Verification items for the finished model (mm, model axes). Face numbers are marked on the shaded views. A direction names the side the tool comes from. Round coordinates to 2 decimals unless told otherwise and drop trailing zeros. Order: outer loops, then holes, each group sorted by start corner. A loop starts at its lowest first (then second) coordinate and runs counter-clockwise, first axis right, second up. Notation, with made-up numbers: (40.25, -38.75) -> (60.25, -38.75) arc R15 cw to (60.25, -31.75) -> close; hole circle Ø2 at (40.25, 18.5). An arc over 180 degrees is marked (long way). Return JSON: item names as keys, results as strings. Group by question number.
Item 1: Access from +Z, -Z, +X, -X, +Y, -Y to the whole of each face (thin tool, end or side, straight path). Record for the marked faces 1, 2 and 3.
Item 2: Draft check along X on the marked faces 4, 5, 6 and 7. Enter one of: pulls with the +X half, pulls with the -X half, needs draft (parallel to the pull), parting line crosses it, or undercut.
Item 3: Sectioned sample at D-D on x = -6.5. Record the cut outline in (y, z), plus the area to 3 significant figures.
Item 4: Scan lines: probe 1 along X at (y, z) = (2, 21); probe 2 along Z at (x, y) = (-6, 4); probe 3 along Z at (x, y) = (8.5, 3.75). Record each from-to range of solid material in increasing order. Write a range as from..to.
Item 5: Sectioned sample at A-A on x = 6. Record the cut outline in (y, z), plus the area to 3 significant figures.
Item 6: Sectioned sample at B-B on y = -1.25. Record the cut outline in (x, z), plus the area to 3 significant figures.
Item 7: Sectioned sample at C-C on x = -3. Record the cut outline in (y, z).
Item 8: Depth check by flat-ended pin: pin 1 Ø2 at (y, z) = (0, 18) entering from +X; pin 2 Ø3.5 at (y, z) = (1, 17.5) entering from -X; pin 3 Ø9 at (x, z) = (-3.5, 4.5) entering from +Y; pin 4 Ø3 at (x, y) = (16, 0.5) entering from +Z. Enter the tip coordinate at first touch or a pass-through.
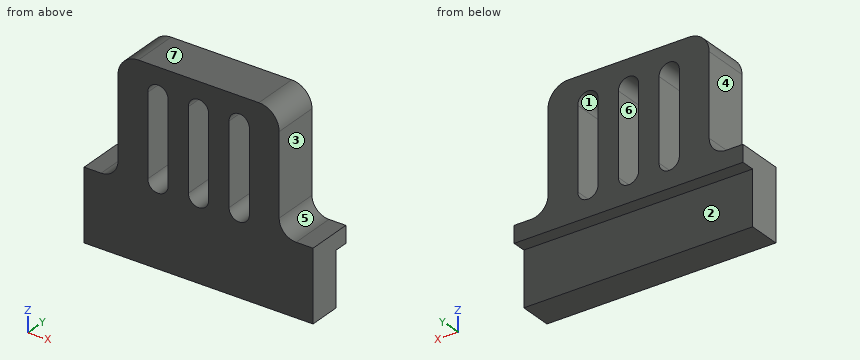
```python
from build123d import *

# Parameters (mm, degrees)
SKETCH_1_W          = 33.8
SKETCH_1_H          = 4.8
EXTRUDE_1_DEPTH     = 28
SKETCH_2_W          = 33.8
SKETCH_2_H          = 2
EXTRUDE_2_DEPTH     = 20
CUT_EXTRUDE_1_DEPTH = 34.404341035
SKETCH_4_W          = 5
SKETCH_4_H          = 17.5
CUT_EXTRUDE_2_DEPTH = 34.404341035
FILLET_1_R          = 3
FILLET_3_R          = 2.5


with BuildPart() as part:
    # 草圖1 → 填料-伸長1 (new body)
    with BuildSketch(Plane.XY):
        Rectangle(SKETCH_1_W, SKETCH_1_H)
    extrude(amount=EXTRUDE_1_DEPTH)

    # 草圖2 → 填料-伸長2 (add)
    with BuildSketch(Plane.XY.offset(28)):
        with Locations((0, 3.4)):
            Rectangle(SKETCH_2_W, SKETCH_2_H)
    extrude(amount=-EXTRUDE_2_DEPTH)

    # 草圖3 → 除料-伸長1 (cut, through all)
    with BuildSketch(Plane(origin=(0, 4.4, 0), x_dir=(1, 0, 0), z_dir=(0, 1, 0))):
        with BuildLine():
            Line((1.5, -12), (1.5, -24))
            ThreePointArc((1.5, -24), (0, -25.5), (-1.5, -24))
            Line((-1.5, -24), (-1.5, -12))
            ThreePointArc((-1.5, -12), (0, -10.5), (1.5, -12))
        make_face()
        with BuildLine():
            Line((7.5, -12), (7.5, -24))
            ThreePointArc((7.5, -24), (6, -25.5), (4.5, -24))
            Line((4.5, -24), (4.5, -12))
            ThreePointArc((4.5, -12), (6, -10.5), (7.5, -12))
        make_face()
        with BuildLine():
            Line((-4.5, -12), (-4.5, -24))
            ThreePointArc((-4.5, -24), (-6, -25.5), (-7.5, -24))
            Line((-7.5, -24), (-7.5, -12))
            ThreePointArc((-7.5, -12), (-6, -10.5), (-4.5, -12))
        make_face()
    extrude(amount=-CUT_EXTRUDE_1_DEPTH, mode=Mode.SUBTRACT)

    # 草圖4 → 除料-伸長2 (cut, through all)
    with BuildSketch(Plane(origin=(0, 4.4, 0), x_dir=(1, 0, 0), z_dir=(0, 1, 0))):
        with Locations((-14.4, -19.25)):
            Rectangle(SKETCH_4_W, SKETCH_4_H)
        with Locations((14.4, -19.25)):
            Rectangle(SKETCH_4_W, SKETCH_4_H)
    extrude(amount=-CUT_EXTRUDE_2_DEPTH, mode=Mode.SUBTRACT)

    # 圓角1
    fillet_1_edges = [part.edges().sort_by_distance(p)[0] for p in [
        (-11.9, 1, 28),
        (11.9, 1, 28),
    ]]
    fillet(fillet_1_edges, radius=FILLET_1_R)

    # 圓角3
    fillet_3_edges = [part.edges().sort_by_distance(p)[0] for p in [
        (-11.9, 1, 10.5),
        (11.9, 1, 10.5),
    ]]
    fillet(fillet_3_edges, radius=FILLET_3_R)


solid = part.part
```
Recorded:
{
 "1": {"face 1": "+Y, -Y", "face 2": "-Z, +X, -X, +Y", "face 3": "+Z, +X, +Y, -Y"},
 "2": {"face 4": "pulls with the -X half", "face 5": "pulls with the +X half", "face 6": "undercut", "face 7": "needs draft"},
 "3": {"outline": "(-2.4, 0) -> (2.4, 0) -> (2.4, 8) -> (4.4, 8) -> (4.4, 10.59) -> (-2.4, 10.59) -> close; (-2.4, 25.41) -> (4.4, 25.41) -> (4.4, 28) -> (-2.4, 28) -> close", "area": "73.6 mm²"},
 "4": {"probe 1": "-11.9..-7.5, -4.5..-1.5, 1.5..4.5, 7.5..11.9", "probe 2": "8..10.5, 25.5..28", "probe 3": "8..28"},
 "5": {"outline": "(-2.4, 0) -> (2.4, 0) -> (2.4, 8) -> (4.4, 8) -> (4.4, 10.5) -> (-2.4, 10.5) -> close; (-2.4, 25.5) -> (4.4, 25.5) -> (4.4, 28) -> (-2.4, 28) -> close", "area": "72.4 mm²"},
 "6": {"outline": "(-16.9, 0) -> (16.9, 0) -> (16.9, 10.5) -> (14.4, 10.5) arc R2.5 cw to (11.9, 13) -> (11.9, 25) arc R3 ccw to (8.9, 28) -> (-8.9, 28) arc R3 ccw to (-11.9, 25) -> (-11.9, 13) arc R2.5 cw to (-14.4, 10.5) -> (-16.9, 10.5) -> close; hole (-7.5, 12) arc R1.5 ccw to (-4.5, 12) -> (-4.5, 24) arc R1.5 ccw to (-7.5, 24) -> close; hole (-1.5, 12) arc R1.5 ccw to (1.5, 12) -> (1.5, 24) arc R1.5 ccw to (-1.5, 24) -> close; hole (4.5, 12) arc R1.5 ccw to (7.5, 12) -> (7.5, 24) arc R1.5 ccw to (4.5, 24) -> close", "area": "641 mm²"},
 "7": {"outline": "(-2.4, 0) -> (2.4, 0) -> (2.4, 8) -> (4.4, 8) -> (4.4, 28) -> (-2.4, 28) -> close"},
 "8": {"pin 1": "x = 11.9", "pin 2": "x = -11.9", "pin 3": "y = 4.4", "pin 4": "z = 10.5"}
}
